from build123d import *

# Parameters (mm, degrees)
CROQUIS1_W                       = 68
CROQUIS1_H                       = 48
BRIDA_BASE1_DEPTH                = 2
BRIDA_DE_ARISTA1_STRIP_W         = 9.4732
BRIDA_DE_ARISTA1_STRIP_H         = 2
BRIDA_DE_ARISTA1_STRIP_CUT_DEPTH = 48
BRIDA_DE_ARISTA1_DEPTH           = 48
BRIDA_DE_ARISTA2_STRIP_W         = 9.4732
BRIDA_DE_ARISTA2_STRIP_H         = 2
BRIDA_DE_ARISTA2_STRIP_CUT_DEPTH = 48
BRIDA_DE_ARISTA2_DEPTH           = 48
DESDOBLAR1_START                 = -121.8089982
DESDOBLAR1_DEPTH                 = 48
DESDOBLAR1_2_DEPTH               = 48
CROQUIS12_W                      = 137.245889802
CROQUIS12_H                      = 40
CORTAR_EXTRUIR1_DEPTH            = 2
DOBLAR1_START                    = -81.8089982
DOBLAR1_DEPTH                    = 8
DOBLAR1_2_DEPTH                  = 8


# Read off the part's stored shape, not the designer's step: Desdoblar1, Doblar1
# Sheet-metal steps are written as plain solids
with BuildPart() as part:
    # Croquis1 → Brida base1 (new body)
    with BuildSketch(Plane.XY.offset(452.5)):
        with Locations((-158.923759138, -97.8089982)):
            Rectangle(CROQUIS1_W, CROQUIS1_H)
    extrude(amount=-BRIDA_BASE1_DEPTH)

    # Brida de arista1 strip (across the edge) → Brida de arista1 strip cut (cut)
    with BuildSketch(Plane(origin=(-192.923759138, -121.8089982, 450.5), x_dir=(1, 0, 0), z_dir=(0, 1, 0))):
        with Locations((-2, -1)):
            Rectangle(BRIDA_DE_ARISTA1_STRIP_W, BRIDA_DE_ARISTA1_STRIP_H)
    extrude(amount=BRIDA_DE_ARISTA1_STRIP_CUT_DEPTH, mode=Mode.SUBTRACT)

    # Brida de arista1 section (across the edge) → Brida de arista1 (add)
    with BuildSketch(Plane(origin=(-192.923759138, -121.8089982, 450.5), x_dir=(1, 0, 0), z_dir=(0, 1, 0))):
        with BuildLine():
            Line((0, 0.7366), (0, 58))
            Line((0, 58), (2, 58))
            Line((2, 58), (2, 0.7366))
            ThreePointArc((2, 0.7366), (2.215745145, 0.215745145), (2.7366, 0))
            Line((2.7366, 0), (2.7366, -2))
            ThreePointArc((2.7366, -2), (0.801531583, -1.198468417), (0, 0.7366))
        make_face()
    extrude(amount=BRIDA_DE_ARISTA1_DEPTH)

    # Brida de arista2 strip (across the edge) → Brida de arista2 strip cut (cut)
    with BuildSketch(Plane(origin=(-192.923759138, -73.8089982, 392.5), x_dir=(0, 0, 1), z_dir=(0, -1, 0))):
        with Locations((-2, -1)):
            Rectangle(BRIDA_DE_ARISTA2_STRIP_W, BRIDA_DE_ARISTA2_STRIP_H)
    extrude(amount=BRIDA_DE_ARISTA2_STRIP_CUT_DEPTH, mode=Mode.SUBTRACT)

    # Brida de arista2 section (across the edge) → Brida de arista2 (add)
    with BuildSketch(Plane(origin=(-192.923759138, -73.8089982, 392.5), x_dir=(0, 0, 1), z_dir=(0, -1, 0))):
        with BuildLine():
            Line((0, 0.7366), (0, 78))
            Line((0, 78), (2, 78))
            Line((2, 78), (2, 0.7366))
            ThreePointArc((2, 0.7366), (2.215745145, 0.215745145), (2.7366, 0))
            Line((2.7366, 0), (2.7366, -2))
            ThreePointArc((2.7366, -2), (0.801531583, -1.198468417), (0, 0.7366))
        make_face()
    extrude(amount=BRIDA_DE_ARISTA2_DEPTH)

    # Desdoblar1 outline → Desdoblar1 (cut)
    with BuildSketch(Plane(origin=(0, 0, 0), x_dir=(1, 0, 0), z_dir=(0, 1, 0)).offset(DESDOBLAR1_START)):
        with BuildLine():
            ThreePointArc((-192.923759138, -449.7634), (-192.898392168, -450.135145906), (-192.822761536, -450.5))
            Line((-192.822761536, -450.5), (-190.187159138, -450.5))
            ThreePointArc((-190.187159138, -450.5), (-190.708013993, -450.284254855), (-190.923759138, -449.7634))
            Line((-190.923759138, -449.7634), (-190.923759138, -395.2366))
            ThreePointArc((-190.923759138, -395.2366), (-191.725290721, -393.301531583), (-193.660359138, -392.5))
            Line((-193.660359138, -392.5), (-270.923759138, -392.5))
            Line((-270.923759138, -392.5), (-270.923759138, -394.5))
            Line((-270.923759138, -394.5), (-193.660359138, -394.5))
            ThreePointArc((-193.660359138, -394.5), (-193.139504283, -394.715745145), (-192.923759138, -395.2366))
            Line((-192.923759138, -395.2366), (-192.923759138, -449.7634))
        make_face()
    extrude(amount=DESDOBLAR1_DEPTH, mode=Mode.SUBTRACT)

    # Desdoblar1 2 outline → Desdoblar1 2 (add)
    with BuildSketch(Plane(origin=(0, 0, 0), x_dir=(1, 0, 0), z_dir=(0, 1, 0)).offset(DESDOBLAR1_START)):
        with BuildLine():
            Line((-327.43304894, -452.5), (-190.187159138, -452.5))
            ThreePointArc((-190.187159138, -452.5), (-191.841426347, -451.943395312), (-192.822761536, -450.5))
            Line((-192.822761536, -450.5), (-327.43304894, -450.5))
            Line((-327.43304894, -450.5), (-327.43304894, -452.5))
        make_face()
    extrude(amount=DESDOBLAR1_2_DEPTH)

    # Croquis12 → Cortar-Extruir1 (cut)
    with BuildSketch(Plane.XY.offset(452.5)):
        with Locations((-258.810104039, -101.8089982)):
            Rectangle(CROQUIS12_W, CROQUIS12_H)
    extrude(amount=-CORTAR_EXTRUIR1_DEPTH, mode=Mode.SUBTRACT)

    # Doblar1 outline → Doblar1 (cut)
    with BuildSketch(Plane(origin=(0, 0, 0), x_dir=(1, 0, 0), z_dir=(0, 1, 0)).offset(DOBLAR1_START)):
        with BuildLine():
            ThreePointArc((-190.187159138, -452.5), (-191.841426347, -451.943395312), (-192.822761536, -450.5))
            Line((-192.822761536, -450.5), (-327.43304894, -450.5))
            Line((-327.43304894, -450.5), (-327.43304894, -452.5))
            Line((-327.43304894, -452.5), (-190.187159138, -452.5))
        make_face()
    extrude(amount=DOBLAR1_DEPTH, mode=Mode.SUBTRACT)

    # Doblar1 2 outline → Doblar1 2 (add)
    with BuildSketch(Plane(origin=(0, 0, 0), x_dir=(1, 0, 0), z_dir=(0, 1, 0)).offset(DOBLAR1_START)):
        with BuildLine():
            Line((-192.923759138, -395.2366), (-192.923759138, -449.7634))
            ThreePointArc((-192.923759138, -449.7634), (-192.898392168, -450.135145906), (-192.822761536, -450.5))
            Line((-192.822761536, -450.5), (-190.187159138, -450.5))
            ThreePointArc((-190.187159138, -450.5), (-190.708013993, -450.284254855), (-190.923759138, -449.7634))
            Line((-190.923759138, -449.7634), (-190.923759138, -395.2366))
            ThreePointArc((-190.923759138, -395.2366), (-191.725290721, -393.301531583), (-193.660359138, -392.5))
            Line((-193.660359138, -392.5), (-270.923759138, -392.5))
            Line((-270.923759138, -392.5), (-270.923759138, -394.5))
            Line((-270.923759138, -394.5), (-193.660359138, -394.5))
            ThreePointArc((-193.660359138, -394.5), (-193.139504283, -394.715745145), (-192.923759138, -395.2366))
        make_face()
    extrude(amount=DOBLAR1_2_DEPTH)


solid = part.part
The listing builds one solid part. Answer for the finished solid, in the listing's coordinates (mm). A direction names the side the tool comes from. Round coordinates to 2 decimals unless told otherwise and drop trailing zeros. Order: outer loops, then holes, each group sorted by start corner. A loop starts at its lowest first (then second) coordinate and runs counter-clockwise, first axis right, second up. Notation, with made-up numbers: (9, 0.25) - (67, 0.25) arc R21 cw to (67, 6.25) - close; hole circle Ø10 at (-12, 1). An arc over 180 degrees is marked (long way). Write item = value, one per line. Start each with the question number.
1) Section A-A, the plane y = -80 is taken. Write down the section's boundary in (x, z).
2) For faces 1 (the flat face through (-192.924, -78, 422)), 2 (the flat face through (-190.924, -78, 423)), 3 (the flat face through (-232, -78, 392.5)), determine the directions among +Z, -Z, +X, -X, +Y, -Y from which every point of the face is accessible in a straight line to the end or side of a thin tool.
3) Section B-B, the plane x = -244.5 is taken. Write down the section's boundary in (y, z).
4) Given pin 1 (1.6 mm diameter, centred on y = -100, z = 451.5, fed in from -X); pin 2 (4 mm diameter, centred on x = -231, y = -76.5, fed in from +Z); pin 3 (4 mm diameter, centred on y = -76.5, z = 419, fed in from -X); pin 4 (3 mm diameter, centred on x = -193, y = -93, fed in from -Z), each flat-ended and moving along its own axis, determine where each tip first touches the part or whether it passes through.
5) Section C-C, the plane z = 410 is taken. Write down the section's boundary in (x, y), plus the area to 3 significant figures.
6) A straight line is drawn through the part: L1, parallel to Z at x = -157, y = -92. Find the intervals that lie inside material, in ascending order.
Results list:
q1.outline = (-270.92, 392.5) - (-193.66, 392.5) arc R2.74 ccw to (-190.92, 395.24) - (-190.92, 449.76) arc R0.74 cw to (-190.19, 450.5) - (-124.92, 450.5) - (-124.92, 452.5) - (-190.19, 452.5) arc R2.74 ccw to (-192.92, 449.76) - (-192.92, 395.24) arc R0.74 cw to (-193.66, 394.5) - (-270.92, 394.5) - close
q2.face_1 = +Z, -X, +Y, -Y
q2.face_2 = -Z, +X, +Y, -Y
q2.face_3 = -Z, +X, -X, +Y, -Y
q3.outline = (-81.81, 392.5) - (-73.81, 392.5) - (-73.81, 394.5) - (-81.81, 394.5) - close
q4.pin_1 = -190.19
q4.pin_2 = 394.5
q4.pin_3 = -192.92
q4.pin_4 = through
q5.outline = (-192.92, -81.81) - (-190.92, -81.81) - (-190.92, -73.81) - (-192.92, -73.81) - close
q5.area = 16.0 mm^2
q6.L1 = 450.5 to 452.5
